Geometry: final body of the model. Coordinates: model frame, mm. Face numbers are marked on the shaded views. A direction names the side the tool comes from. Coordinates: 2 decimals unless noted, no trailing zeros. Order: outer loops, then holes, each group sorted by start corner. A loop starts at its lowest first (then second) coordinate and runs counter-clockwise, first axis right, second up. Notation, with made-up numbers: M 30,-9.75 L 42,-9.75 A17 ccw 42,20.25 Z; hole C 36,22 d5. An arc over 180 degrees is marked long. Use CSV: the item, a comma, the result in double quotes. Start each with the question number.
Q1. Access query for the marked faces 1, 2 and 3. Directions: +Z, -Z, +X, -X, +Y, -Y. A direction counts if a zero-diameter tool reaches every point of the face in a straight line with its end or side. Return the directions, or none.
Q2. Ray query, probe 1 along Y at (x, z) = (0, 4.5); probe 2 along Z at (x, y) = (-2.5, -5); probe 3 along X at (y, z) = (0, -7.5). Return the intervals inside material, ascending.
Q3. Section query A-A, the plane z = 12.5. Output: boundary loops of the cut face in (x, y), and give its area (3 significant figures).
Q4. Mould query, pull axis Y, two halves, no side actions, for the marked faces 4, 5, 6 and 7. Classes: +Y half, -Y half, draft (parallel to the pull), parting line (faces both ways), or undercut.
Q5. First-contact query: P1, Ø10, axis at y = 0.5, z = -5.5, coming from the +X side; P2, Ø7, axis at x = 18, y = -19.5, coming from the -Z side; P3, Ø1.5, axis at x = -5.5, z = -13.5, coming from the +Y side. Flat tips, straight axial feed; report the tip coordinate or a pass-through.
Q6. Section query D-D, the plane z = -1. Output: boundary loops of the cut face in (x, y), and give its area (3 significant figures).
from build123d import *

# Parameters (mm, degrees)
F2_R      = 26.134352
F3_DEPTH  = 0.635
F5_DEPTH  = 4.064
F6_R      = 3.429
F7_DEPTH  = 25.4
F8_R      = 26.035
F9_DEPTH  = 0.635
F10_R     = 7.873192
F10_R_2   = 7.315587
F11_DEPTH = 22.86
F12_R     = 31.75
F13_DEPTH = 25.4


with BuildPart() as f1:
    # F0 (on Front) → F1 (revolve)
    with BuildSketch(Plane.XZ):
        Polygon((0, 21.606712), (0, 0), (7.874, 0), (25.908, 5.858712), (25.908, 21.606712), align=None)
    revolve(axis=Axis((0, 0, 10.803356), (0, 0, -1)))

    # F2 (on face) → F3 (cut)
    with BuildSketch(Plane.XY.offset(21.606712)):
        Circle(F2_R)
    extrude(amount=-F3_DEPTH, mode=Mode.SUBTRACT)

    # F4 (on face) → F5 (cut)
    with BuildSketch(Plane.XY.offset(20.971712)):
        Polygon((2.242883, -6.128247), (6.428659, -1.12173), (4.185776, 5.006517), (-2.242883, 6.128247), (-6.428659, 1.12173), (-4.185776, -5.006517), align=None)
    extrude(amount=-F5_DEPTH, mode=Mode.SUBTRACT)

    # F6 (on face) → F7 (cut)
    with BuildSketch(Plane.XY.offset(16.907712)):
        Circle(F6_R)
    extrude(amount=-F7_DEPTH, mode=Mode.SUBTRACT)

    # F8 (on face) → F9 (join)
    with BuildSketch(Plane.XY.offset(20.971712)):
        Circle(F8_R)
    extrude(amount=F9_DEPTH)

    # F10 (on face) → F11 (join)
    with BuildSketch(Plane(origin=(0, 0, 0), x_dir=(1, 0, 0), z_dir=(0, 0, -1))):
        Circle(F10_R)
        Circle(F10_R_2, mode=Mode.SUBTRACT)
    extrude(amount=F11_DEPTH)

    # F12 (on face) → F13 (cut)
    with BuildSketch(Plane.XY.offset(21.606712)):
        with Locations((-50.8, 0)):
            Circle(F12_R)
        with Locations((0, 50.8)):
            Circle(F12_R)
        with Locations((50.8, 0)):
            Circle(F12_R)
        with Locations((0, -50.8)):
            Circle(F12_R)
    extrude(amount=-F13_DEPTH, mode=Mode.SUBTRACT)


solid = f1.part
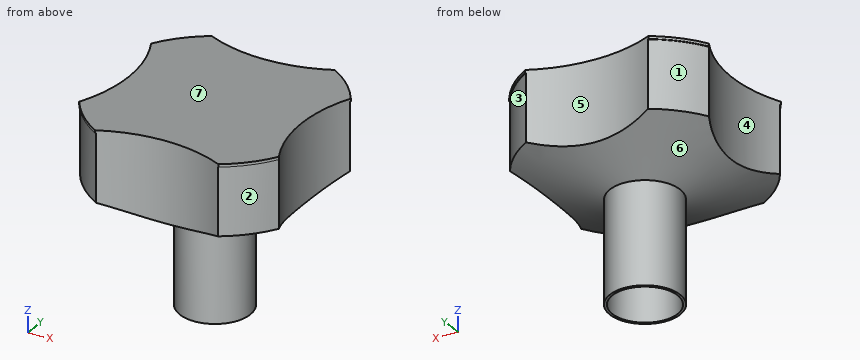
Responses:
1,face 1,"-Z, -X, +Y"
1,face 2,"-Z, +X, -Y"
1,face 3,"-Z, +X, +Y"
2,probe 1,"y = -19.05 to -3.43, 3.43 to 19.05"
2,probe 2,"z = 0 to 16.91, 20.97 to 21.61"
2,probe 3,"x = -7.87 to -7.32, 7.32 to 7.87"
3,outline,"M -22.08,-13.55 A25.91 ccw -13.55,-22.08 A31.75 cw 13.55,-22.08 A25.91 ccw 22.08,-13.55 A31.75 cw 22.08,13.55 A25.91 ccw 13.55,22.08 A31.75 cw -13.55,22.08 A25.91 ccw -22.08,13.55 A31.75 cw Z; hole C 0,0 d6.86"
3,area,"1,570 mm²"
4,face 4,"undercut"
4,face 5,"+Y half"
4,face 6,"parting line"
4,face 7,"draft"
5,P1,"stops at x = 7.87"
5,P2,"stops at z = 4.93"
5,P3,"stops at y = 6.28"
6,outline,"C 0,0 d15.75; hole C 0,0 d14.63"
6,area,"26.6 mm²"
